Model file for the job. Use its own axes, mm. Face numbers are marked on the shaded views. Give positions to 0.01 mm unless a question says otherwise; leave off trailing zeros. Write each loop counter-clockwise with the first axis right and the second up, starting at its lowest first coordinate (ties: lowest second). Pieces come first, ordered by that corner, then holes. Notation, with made-up numbers: (18, 7.25) - (59, 7.25) arc R30 cw to (59, 33.25) - close; hole circle Ø9 at (47.5, -28.5). An arc over 180 degrees is marked (long way). Use a Markdown table: item, result. Add a question column.
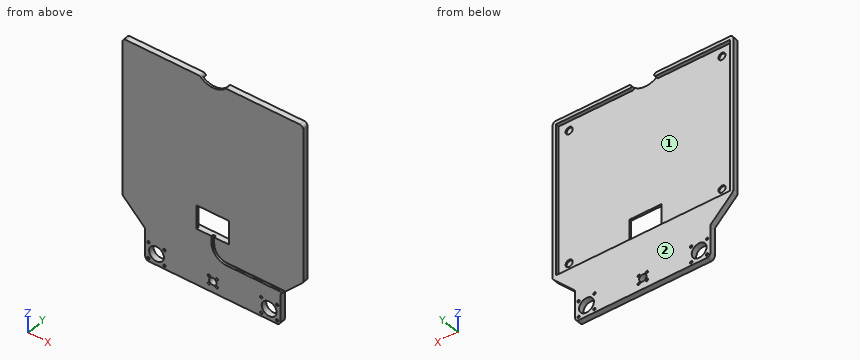
```python
from build123d import *
from OCP.BRepFilletAPI import BRepFilletAPI_MakeFillet

# Parameters (mm, degrees)
SALIENTE_EXTRUIR1_DEPTH = 8
REDONDEO1_R1            = 7
REDONDEO1_R2            = 5
REDONDEO1_R3            = 5
CROQUIS17_R             = 5.15
CROQUIS17_R_2           = 1.75
CORTAR_EXTRUIR15_DEPTH  = 316.011904537
CROQUIS18_R             = 1.75
CORTAR_EXTRUIR16_DEPTH  = 316.011904537
CROQUIS19_R             = 1.75
CORTAR_EXTRUIR17_DEPTH  = 316.011904537
CROQUIS20_R             = 1.75
CORTAR_EXTRUIR18_DEPTH  = 316.011904537
CROQUIS21_R             = 1.75
CORTAR_EXTRUIR19_DEPTH  = 316.011904537
CROQUIS22_R             = 10.55
CORTAR_EXTRUIR20_DEPTH  = 316.011904537
CROQUIS23_R             = 1.75
CORTAR_EXTRUIR21_DEPTH  = 316.011904537
CROQUIS24_R             = 1.75
CORTAR_EXTRUIR22_DEPTH  = 316.011904537
CROQUIS25_R             = 1.75
CORTAR_EXTRUIR23_DEPTH  = 316.011904537
CROQUIS26_R             = 1.75
CORTAR_EXTRUIR24_DEPTH  = 316.011904537
CROQUIS27_R             = 10.55
CORTAR_EXTRUIR25_DEPTH  = 316.011904537
CROQUIS31_W             = 247
CROQUIS31_H             = 217.984697531
CORTAR_EXTRUIR29_DEPTH  = 5
CROQUIS32_R             = 5.1
CORTAR_EXTRUIR30_DEPTH  = 2
CORTAR_EXTRUIR31_DEPTH  = 3
CORTAR_EXTRUIR32_REACH  = 317.012
CROQUIS34_R             = 25
REDONDEO4_R             = 2


with BuildPart() as part:
    # Croquis1 → Saliente-Extruir1 (new body)
    with BuildSketch(Plane(origin=(0, 4, 0), x_dir=(1, 0, 0), z_dir=(0, 1, 0))):
        Polygon((96, 16), (-96, 16), (-96, -29), (-128.5, -61.623586062), (-128.5, -287.5), (128.5, -287.5), (128.5, -61.623586062), (96, -29), align=None)
    extrude(amount=-SALIENTE_EXTRUIR1_DEPTH)

    # Redondeo1: one fillet with a radius per group of edges: ONE call of the kernel's fillet builder (fillet() takes one radius for all edges)
    redondeo1_edges_1 = [part.edges().sort_by_distance(p)[0] for p in [
        (-128.5, 0, 61.623586062),
        (128.5, 0, 61.623586062),
    ]]
    redondeo1_edges_2 = [part.edges().sort_by_distance(p)[0] for p in [
        (96, 0, -16),
        (-96, 0, 29),
        (-96, 0, -16),
        (96, 0, 29),
    ]]
    redondeo1_edges_3 = [part.edges().sort_by_distance(p)[0] for p in [
        (128.5, 0, 287.5),
        (-128.5, 0, 287.5),
    ]]
    redondeo1 = BRepFilletAPI_MakeFillet(part.part.solid().wrapped)
    for e in redondeo1_edges_1:
        redondeo1.Add(REDONDEO1_R1, e.wrapped)
    for e in redondeo1_edges_2:
        redondeo1.Add(REDONDEO1_R2, e.wrapped)
    for e in redondeo1_edges_3:
        redondeo1.Add(REDONDEO1_R3, e.wrapped)
    add(Compound.cast(redondeo1.Shape()), mode=Mode.REPLACE)

    # Croquis17 → Cortar-Extruir15 (cut, through all)
    with BuildSketch(Plane.XZ.offset(4)):
        with Locations(Location((0, -0.1, 0), (0, 0, 90))):
            Circle(CROQUIS17_R)
        with Locations(Location((-5.656854249, -5.756854249, 0), (0, 0, 270))):
            Circle(CROQUIS17_R_2)
        with Locations(Location((5.656854249, -5.756854249, 0), (0, 0, 270))):
            Circle(CROQUIS17_R_2)
        with Locations(Location((5.656854249, 5.556854249, 0), (0, 0, 270))):
            Circle(CROQUIS17_R_2)
        with Locations(Location((-5.656854249, 5.556854249, 0), (0, 0, 270))):
            Circle(CROQUIS17_R_2)
    extrude(amount=-CORTAR_EXTRUIR15_DEPTH, mode=Mode.SUBTRACT)

    # Croquis18 → Cortar-Extruir16 (cut, through all)
    with BuildSketch(Plane.XZ.offset(4)):
        with Locations(Location((91.313708499, 11.313708499, 0), (0, 0, 90))):
            Circle(CROQUIS18_R)
    extrude(amount=-CORTAR_EXTRUIR16_DEPTH, mode=Mode.SUBTRACT)

    # Croquis19 → Cortar-Extruir17 (cut, through all)
    with BuildSketch(Plane.XZ.offset(4)):
        with Locations(Location((91.313708499, -11.313708499, 0), (0, 0, 90))):
            Circle(CROQUIS19_R)
    extrude(amount=-CORTAR_EXTRUIR17_DEPTH, mode=Mode.SUBTRACT)

    # Croquis20 → Cortar-Extruir18 (cut, through all)
    with BuildSketch(Plane.XZ.offset(4)):
        with Locations(Location((68.686291501, 11.313708499, 0), (0, 0, 90))):
            Circle(CROQUIS20_R)
    extrude(amount=-CORTAR_EXTRUIR18_DEPTH, mode=Mode.SUBTRACT)

    # Croquis21 → Cortar-Extruir19 (cut, through all)
    with BuildSketch(Plane.XZ.offset(4)):
        with Locations(Location((68.686291501, -11.313708499, 0), (0, 0, 90))):
            Circle(CROQUIS21_R)
    extrude(amount=-CORTAR_EXTRUIR19_DEPTH, mode=Mode.SUBTRACT)

    # Croquis22 → Cortar-Extruir20 (cut, through all)
    with BuildSketch(Plane.XZ.offset(4)):
        with Locations(Location((80, 0, 0), (0, 0, 90))):
            Circle(CROQUIS22_R)
    extrude(amount=-CORTAR_EXTRUIR20_DEPTH, mode=Mode.SUBTRACT)

    # Croquis23 → Cortar-Extruir21 (cut, through all)
    with BuildSketch(Plane.XZ.offset(4)):
        with Locations(Location((-68.686291501, -11.313708499, 0), (0, 0, 90))):
            Circle(CROQUIS23_R)
    extrude(amount=-CORTAR_EXTRUIR21_DEPTH, mode=Mode.SUBTRACT)

    # Croquis24 → Cortar-Extruir22 (cut, through all)
    with BuildSketch(Plane.XZ.offset(4)):
        with Locations(Location((-68.686291501, 11.313708499, 0), (0, 0, 90))):
            Circle(CROQUIS24_R)
    extrude(amount=-CORTAR_EXTRUIR22_DEPTH, mode=Mode.SUBTRACT)

    # Croquis25 → Cortar-Extruir23 (cut, through all)
    with BuildSketch(Plane.XZ.offset(4)):
        with Locations(Location((-91.313708499, 11.313708499, 0), (0, 0, 90))):
            Circle(CROQUIS25_R)
    extrude(amount=-CORTAR_EXTRUIR23_DEPTH, mode=Mode.SUBTRACT)

    # Croquis26 → Cortar-Extruir24 (cut, through all)
    with BuildSketch(Plane.XZ.offset(4)):
        with Locations(Location((-91.313708499, -11.313708499, 0), (0, 0, 90))):
            Circle(CROQUIS26_R)
    extrude(amount=-CORTAR_EXTRUIR24_DEPTH, mode=Mode.SUBTRACT)

    # Croquis27 → Cortar-Extruir25 (cut, through all)
    with BuildSketch(Plane.XZ.offset(4)):
        with Locations(Location((-80, 0, 0), (0, 0, 90))):
            Circle(CROQUIS27_R)
    extrude(amount=-CORTAR_EXTRUIR25_DEPTH, mode=Mode.SUBTRACT)

    # Croquis31 → Cortar-Extruir29 (cut)
    with BuildSketch(Plane(origin=(0, 4, 0), x_dir=(1, 0, 0), z_dir=(0, 1, 0))):
        with Locations((0, -173.507651235)):
            Rectangle(CROQUIS31_W, CROQUIS31_H)
    extrude(amount=-CORTAR_EXTRUIR29_DEPTH, mode=Mode.SUBTRACT)

    # Croquis32 → Cortar-Extruir30 (cut)
    with BuildSketch(Plane(origin=(0, -1, 0), x_dir=(1, 0, 0), z_dir=(0, 1, 0))):
        with Locations(Location((-108.504553774, -77.749220728, 0), (0, 0, 270))):
            Circle(CROQUIS32_R)
        with Locations(Location((-108.504553774, -269.266081741, 0), (0, 0, 270))):
            Circle(CROQUIS32_R)
        with Locations(Location((108.504553774, -269.266081741, 0), (0, 0, 270))):
            Circle(CROQUIS32_R)
        with Locations(Location((108.504553774, -77.749220728, 0), (0, 0, 270))):
            Circle(CROQUIS32_R)
    extrude(amount=-CORTAR_EXTRUIR30_DEPTH, mode=Mode.SUBTRACT)

    # Croquis33 → Cortar-Extruir31 (cut)
    with BuildSketch(Plane(origin=(0, -1, 0), x_dir=(1, 0, 0), z_dir=(0, 1, 0))):
        Polygon((-23, -98.515302469), (23, -98.515302469), (23, -64.515302469), (2, -64.515302469), (-2, -64.515302469), (-23, -64.515302469), align=None)
        with BuildLine():
            Line((-2, -64.515302469), (2, -64.515302469))
            Line((2, -64.515302469), (2, -54.515302469))
            ThreePointArc((2, -54.515302469), (7.272077939, -41.787380408), (20, -36.515302469))
            Line((20, -36.515302469), (103.48683268, -36.515302469))
            Line((103.48683268, -36.515302469), (99.50198565, -32.515302469))
            Line((99.50198565, -32.515302469), (20, -32.515302469))
            ThreePointArc((20, -32.515302469), (4.443650814, -38.958953283), (-2, -54.515302469))
            Line((-2, -54.515302469), (-2, -64.515302469))
        make_face()
    extrude(amount=-CORTAR_EXTRUIR31_DEPTH, mode=Mode.SUBTRACT)

    # Croquis34 → Cortar-Extruir32 (cut, up to next)
    with BuildSketch(Plane(origin=(0, 4, 0), x_dir=(1, 0, 0), z_dir=(0, 1, 0)), mode=Mode.PRIVATE) as cortar_extruir32_sk1:
        with Locations((0, -304.5)):
            Circle(CROQUIS34_R)
    cortar_extruir32_tool1 = extrude(cortar_extruir32_sk1.sketch, amount=-CORTAR_EXTRUIR32_REACH, mode=Mode.PRIVATE) & part.part
    add(cortar_extruir32_tool1.solids().sort_by_distance((0, 4, 304.5))[0], mode=Mode.SUBTRACT)

    # Redondeo4
    redondeo4_edges = [part.edges().sort_by_distance(p)[0] for p in [
        (11.874342087, 1.5, 282.5),
        (-11.874342087, 1.5, 282.5),
        (18.33030278, 0, 287.5),
        (-18.33030278, 0, 287.5),
    ]]
    fillet(redondeo4_edges, radius=REDONDEO4_R)


solid = part.part
```
(1) Band-saw the part on D-D (x = 38). Write the cut outline in (y, z), then the cut area to 3 significant figures.
(2) Band-saw the part on C-C (z = 141). Write the cut outline in (x, y).
(3) Band-saw the part on A-A (x = 80). Write the cut outline in (y, z), then the cut area to 3 significant figures.
(4) Flat gauge pins, fed straight in: pin 1 (2.5 mm diameter, centred on y = -2.5, z = 62, fed in from -X); pin 2 (8 mm diameter, centred on x = -108.5, z = 77.75, fed in from +Y). Where does each tip first touch, or does it go through?
(5) Band-saw the part on B-B (z = 0). Write the cut outline in (x, y).
(6) Two-plate mould, pull along Z, no slides. Class the marked faces 1 and 2: +Z half, -Z half, draft (parallel to the pull), parting line (faces both ways), or undercut.
(7) Probe probe 1 along Z at (x, y) = (75.5, 3); probe 2 along X at (y, z) = (-1.25, 77); probe 3 along Z at (x, y) = (48.5, 2.75). List the from-to ranges inside material, lowest first. Write a range as [from, to].
Model answer:
| question | item | result |
|---|---|---|
| 1 | outline | (-4, -16) - (4, -16) - (4, 64.52) - (-1, 64.52) - (-1, 282.5) - (4, 282.5) - (4, 287.5) - (-4, 287.5) - (-4, 36.52) - (-1, 36.52) - (-1, 32.52) - (-4, 32.52) - close |
| 1 | area | 1,330 mm^2 |
| 2 | outline | (-128.5, -4) - (128.5, -4) - (128.5, 4) - (123.5, 4) - (123.5, -1) - (-123.5, -1) - (-123.5, 4) - (-128.5, 4) - close |
| 3 | outline | (-4, -16) - (4, -16) - (4, -10.55) - (-4, -10.55) - close; (-4, 10.55) - (4, 10.55) - (4, 64.52) - (-1, 64.52) - (-1, 282.5) - (4, 282.5) - (4, 287.5) - (-4, 287.5) - (-4, 36.52) - (-1, 36.52) - (-1, 32.52) - (-4, 32.52) - close |
| 3 | area | 1,160 mm^2 |
| 4 | pin 1 | stops at x = -128.38 |
| 4 | pin 2 | stops at y = -3 |
| 5 | outline | (-96, -4) - (-90.55, -4) - (-90.55, 4) - (-96, 4) - close; (-69.45, -4) - (-5.15, -4) - (-5.15, 4) - (-69.45, 4) - close; (5.15, -4) - (69.45, -4) - (69.45, 4) - (5.15, 4) - close; (90.55, -4) - (96, -4) - (96, 4) - (90.55, 4) - close |
| 6 | face 1 | undercut |
| 6 | face 2 | draft |
| 7 | probe 1 | z = [-16, -9.54], [9.54, 64.52], [282.5, 287.5] |
| 7 | probe 2 | x = [-128.5, -113.55], [-103.46, -23], [23, 103.46], [113.55, 128.5] |
| 7 | probe 3 | z = [-16, 64.52], [282.5, 287.5] |
